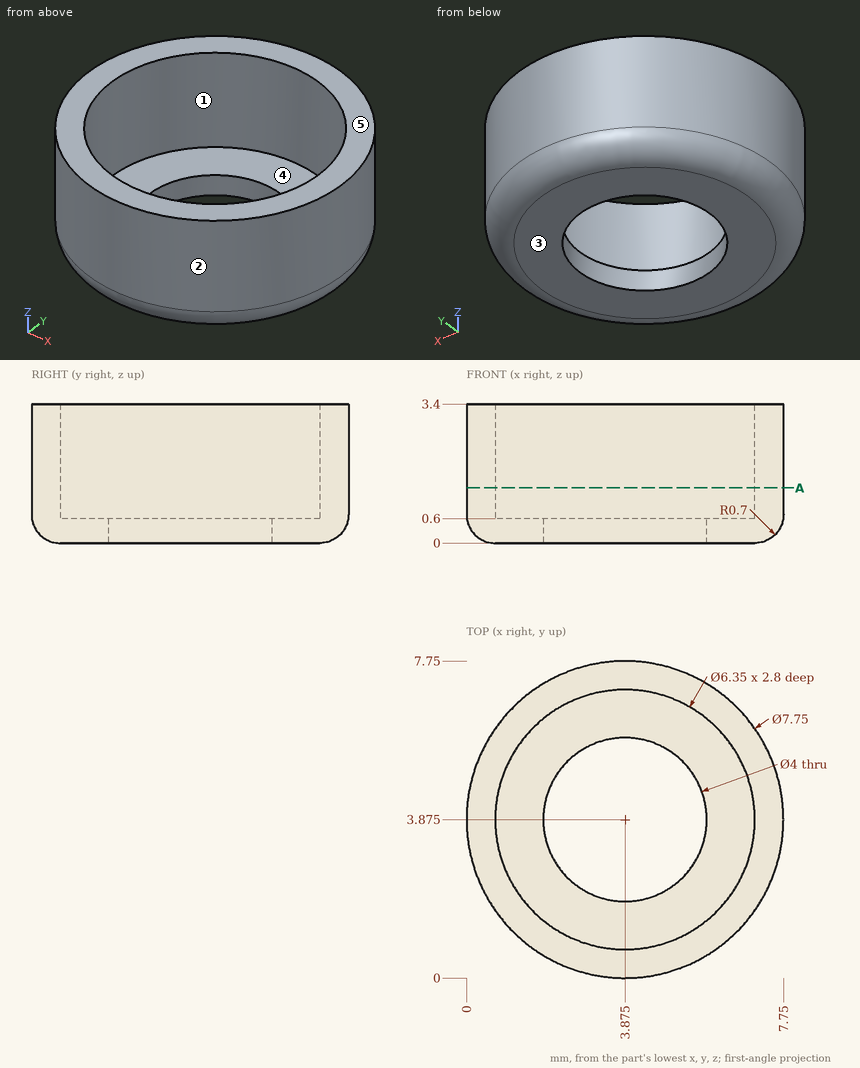
Design review of the part shown in the three views and the two pictorial views. Dimensions are in mm from the part's minimum x, y and z. A direction names the side the tool comes from. Give positions to 0.01 mm unless a question says otherwise; leave off trailing zeros. Order: outer loops, then holes, each group sorted by start corner. A loop starts at its lowest first (then second) coordinate and runs counter-clockwise, first axis right, second up. Notation, with made-up numbers: M -31,-40 L -15,-40 A14 ccw -15,-33 Z; hole C 37,80.5 d1. An arc over 180 degrees is marked long. Answer in a Markdown table with one row per item. Add a question column.
(1) For pin 1 (2.5 mm diameter, centred on x = 3.875, y = 3.875, fed in from -Z); pin 2 (1 mm diameter, centred on y = 4.5, z = 3, fed in from +X); pin 3 (2 mm diameter, centred on x = 6, z = 1, fed in from +Y); pin 4 (1.5 mm diameter, centred on x = 3.5, y = 7, fed in from -Z), all flat-tipped, find the tip position at first contact; note any pin that passes through.
(2) Mouldability with a two-part tool opening along Y and no side actions: class the marked faces 1, 2 and 3 as +Y half, -Y half, draft (parallel to the pull), parting line (faces both ways), or undercut.
(3) Wall thickness on probe 1 along Y at (x, z) = (4, 1.9); probe 2 along Z at (x, y) = (1.25, 3.5); probe 3 along X at (y, z) = (5.25, 1.3): over which ranges is each line inside the solid? List them lowest first. Write a range as [from, to].
(4) For the marked faces 4 and 5, list the 3-axis set-ups (+Z, -Z, +X, -X, +Y, -Y) from which the entire face can be reached by the end or side of a thin tool; tool diameter is ignored.
(5) Consider section A-A on z = 1.35. State the section outline as (x, y) points (3 decimals), and give its area (3 significant figures).
Evaluation:
| question | item | result |
|---|---|---|
| 1 | pin 1 | passes through |
| 1 | pin 2 | stops at x = 7.75 |
| 1 | pin 3 | stops at y = 7.58 |
| 1 | pin 4 | stops at z = 0 |
| 2 | face 1 | undercut |
| 2 | face 2 | parting line |
| 2 | face 3 | draft |
| 3 | probe 1 | y = [0, 0.7], [7.05, 7.75] |
| 3 | probe 2 | z = [0, 0.6] |
| 3 | probe 3 | x = [0.25, 1.01], [6.74, 7.5] |
| 4 | face 4 | +Z |
| 4 | face 5 | +Z, +X, -X, +Y, -Y |
| 5 | outline | C 3.875,3.875 d7.75; hole C 3.875,3.875 d6.35 |
| 5 | area | 15.5 mm^2 |
